```python
from build123d import *

# Parameters (mm, degrees)
SKETCH2_R      = 6.985
EXTRUDE1_DEPTH = 7.112
SKETCH3_R      = 0.3556
EXTRUDE2_DEPTH = 7.62
SKETCH4_R      = 1.397
EXTRUDE3_DEPTH = 3.81


with BuildPart() as part:
    # Sketch2 → Extrude1 (new body)
    with BuildSketch(Plane(origin=(0, 0, 0), x_dir=(1, 0, 0), z_dir=(0, 1, 0))):
        with Locations(Location((0, 0, 0), (0, 0, 270))):
            Circle(SKETCH2_R)
    extrude(amount=EXTRUDE1_DEPTH)

    # Sketch3 → Extrude2 (add)
    with BuildSketch(Plane.XZ):
        with Locations(Location((3.683, 0, 0), (0, 0, 90))):
            Circle(SKETCH3_R)
        with Locations(Location((-3.683, 0, 0), (0, 0, 90))):
            Circle(SKETCH3_R)
    extrude(amount=EXTRUDE2_DEPTH)

    # Sketch4 → Extrude3 (cut)
    with BuildSketch(Plane(origin=(0, 7.112, 0), x_dir=(1, 0, 0), z_dir=(0, 1, 0))):
        with Locations(Location((0, 0, 0), (0, 0, 270))):
            Circle(SKETCH4_R)
    extrude(amount=-EXTRUDE3_DEPTH, mode=Mode.SUBTRACT)


solid = part.part
```
Model file for the job. Use its own axes, mm. Coordinates: 2 decimals unless noted, no trailing zeros. Write each loop counter-clockwise with the first axis right and the second up, starting at its lowest first coordinate (ties: lowest second). Pieces come first, ordered by that corner, then holes. Notation, with made-up numbers: (-16.5, 39) - (-1.5, 39) arc R18 ccw to (-1.5, 56) - close; hole circle Ø8 at (-30, 10.5). An arc over 180 degrees is marked (long way). One line per question, with ' | ' between items. Start each with the question number.
Q1. Drill centre lines: line 1 (X direction, y = 6.25, z = 0) (3 decimals); line 2 (Y direction, x = -3, z = -0.5); line 3 (Z direction, x = 4, y = 1.5). Where is each one in solid material? Low to high. Write a range as [from, to].
Q2. Cut at A-A, the plane x = 0. List the corners of the cut face in (y, z) (3 decimals), then the cut area to 3 significant figures.
Q3. Cut at D-D, the plane y = -6. List the corners of the cut face in (x, z), then the cut area to 3 significant figures.
Q4. Pin check, flat tips, straight feed: pin 1 (1.5 mm diameter, centred on y = -0.5, z = 2, fed in from +X); pin 2 (3 mm diameter, centred on x = 0, z = 0, fed in from -Y); pin 3 (1 mm diameter, centred on x = -3, y = -2, fed in from +Z); pin 4 (2 mm diameter, centred on x = -2, y = -5, fed in from -Z). Stop position of each tip, or through.
Q5. Pull direction Z, two halves, no side cores. Call faces 1 (the face through (2, 7.112, 0)), 2 (the face through (0, 3.302, 0)), 3 (the face through (6.926, 3.506, -0.909)): pulls with the +Z half, pulls with the -Z half, needs draft (parallel to the pull), parting line crosses it, or undercut.
Q6. Cut at B-B, the plane z = 0. List the corners of the cut face in (x, y) (3 decimals).
Q7. Cut at C-C, the plane y = 6. List the corners of the cut face in (x, z) (3 decimals), then the cut area to 3 significant figures.
Answer below:
1) line 1: [-6.985, -1.397], [1.397, 6.985] | line 2: [0, 7.11] | line 3: [-5.73, 5.73]
2) outline: (0, -6.985) - (7.112, -6.985) - (7.112, -1.397) - (3.302, -1.397) - (3.302, 1.397) - (7.112, 1.397) - (7.112, 6.985) - (0, 6.985) - close | area: 88.7 mm^2
3) outline: circle Ø0.71 at (-3.68, 0); circle Ø0.71 at (3.68, 0) | area: 0.795 mm^2
4) pin 1: x = 6.83 | pin 2: y = 0 | pin 3: z = 0.3 | pin 4: through
5) face 1: needs draft | face 2: undercut | face 3: parting line crosses it
6) outline: (-6.985, 0) - (-4.039, 0) - (-4.039, -7.62) - (-3.327, -7.62) - (-3.327, 0) - (3.327, 0) - (3.327, -7.62) - (4.039, -7.62) - (4.039, 0) - (6.985, 0) - (6.985, 7.112) - (1.397, 7.112) - (1.397, 3.302) - (-1.397, 3.302) - (-1.397, 7.112) - (-6.985, 7.112) - close
7) outline: circle Ø13.97 at (0, 0); hole circle Ø2.794 at (0, 0) | area: 147 mm^2
